Job drawing, mm, ordinate dimensions from the low corner. One solid piece. A direction names the side the tool comes from. Round coordinates to 2 decimals unless told otherwise and drop trailing zeros. Write each loop counter-clockwise with the first axis right and the second up, starting at its lowest first coordinate (ties: lowest second). Pieces come first, ordered by that corner, then holes. Notation, with made-up numbers: M 50,-10.75 L 108,-10.75 A20 cw 108,12.25 Z; hole C 11.25,68 d7. An arc over 180 degrees is marked long. One line per item, written item: value. Start each with the question number.
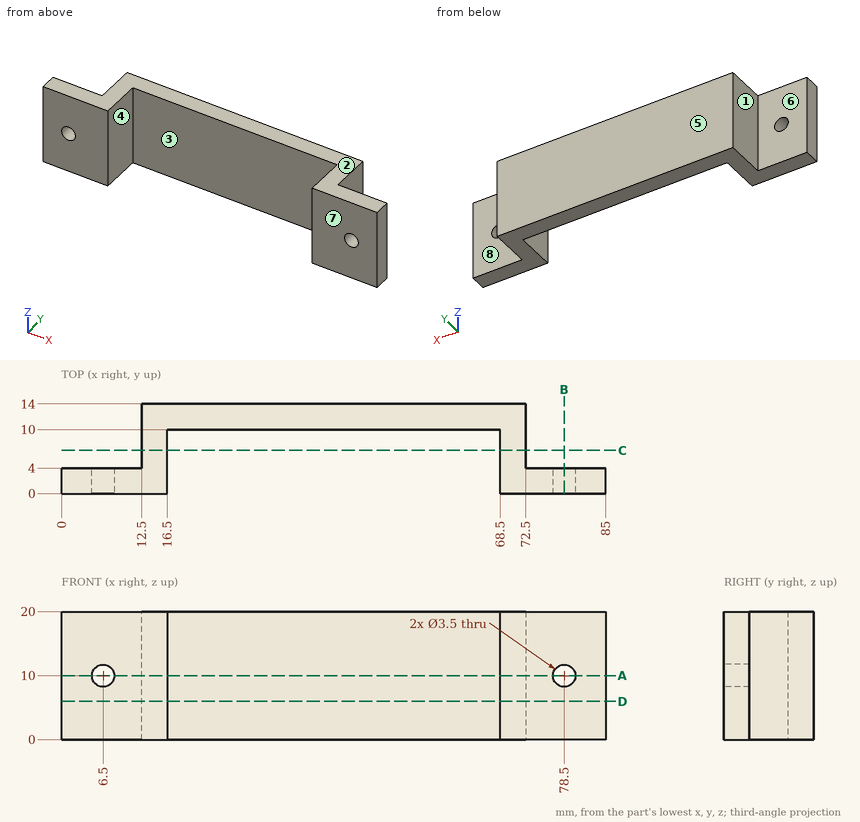
Item 1: Drill centre lines: line 1 (X direction, y = 1, z = 17.5); line 2 (Z direction, x = 6.5, y = 1.5); line 3 (X direction, y = 5.75, z = 3). Where is each one in solid material? Low to high.
Item 2: Cut at A-A, the plane z = 10. Write the cut outline in (x, y).
Item 3: Drop flat-ended pins along their axis: pin 1 (6 mm diameter, centred on x = 52.5, z = 10, fed in from -Y); pin 2 (4 mm diameter, centred on x = 77.5, z = 11.5, fed in from +Y); pin 3 (8 mm diameter, centred on y = 11, z = 5.5, fed in from +X); pin 4 (3 mm diameter, centred on x = 6.5, z = 10, fed in from +Y). Give the stop position or say it passes through.
Item 4: Which spindle directions (+Z, -Z, +X, -X, +Y, -Y) get a long thin tool onto all of the face, cutting with end or side? Do the marked faces 4, 5, 6, 7 and 8. Say none if no direction does.
Item 5: Cut at D-D, the plane z = 6. Write the cut outline in (x, y), plus the area to 3 significant figures.
Item 6: Two-plate mould, pull along X, no slides. Class the marked faces 1, 2 and 3: pulls with the +X half, pulls with the -X half, needs draft (parallel to the pull), parting line crosses it, or undercut.
Item 7: Cut at B-B, the plane x = 78.5. Write the cut outline in (y, z).
Item 8: Cut at C-C, the plane y = 6.75. Write the cut outline in (x, z), plus the area to 3 significant figures.
Computed values:
1. line 1: x = 0 to 16.5, 68.5 to 85
1. line 2: z = 0 to 8.25, 11.75 to 20
1. line 3: x = 12.5 to 16.5, 68.5 to 72.5
2. outline: M 0,0 L 4.75,0 L 4.75,4 L 0,4 Z; M 8.25,0 L 16.5,0 L 16.5,10 L 68.5,10 L 68.5,0 L 76.75,0 L 76.75,4 L 72.5,4 L 72.5,14 L 12.5,14 L 12.5,4 L 8.25,4 Z; M 80.25,0 L 85,0 L 85,4 L 80.25,4 Z
3. pin 1: stops at y = 10
3. pin 2: stops at y = 4
3. pin 3: stops at x = 72.5
3. pin 4: passes through
4. face 4: +Z, -Z, -Y
4. face 5: +Z, -Z, +X, -X, +Y
4. face 6: +Z, -Z, -X, +Y
4. face 7: +Z, -Z, +X, -X, -Y
4. face 8: +Z, -Z, +X, +Y
5. outline: M 0,0 L 16.5,0 L 16.5,10 L 68.5,10 L 68.5,0 L 85,0 L 85,4 L 72.5,4 L 72.5,14 L 12.5,14 L 12.5,4 L 0,4 Z
5. area: 420 mm2
6. face 1: pulls with the -X half
6. face 2: needs draft
6. face 3: undercut
7. outline: M 0,0 L 4,0 L 4,8.25 L 0,8.25 Z; M 0,11.75 L 4,11.75 L 4,20 L 0,20 Z
8. outline: M 12.5,0 L 16.5,0 L 16.5,20 L 12.5,20 Z; M 68.5,0 L 72.5,0 L 72.5,20 L 68.5,20 Z
8. area: 160 mm2
